from build123d import *

# Parameters (mm, degrees)
SKETCH_1_W               = 55
SKETCH_1_H               = 55
EXTRUDE_1_DEPTH          = 10
SKETCH_2_R               = 17.5
EXTRUDE_2_DEPTH          = 1
SKETCH_3_R               = 16.25
EXTRUDE_3_DEPTH          = 2
SKETCH_4_R               = 17.5
EXTRUDE_4_DEPTH          = 1
SKETCH_5_R               = 4.25
CUT_EXTRUDE_1_DEPTH      = 3
SKETCH_6_R               = 2.5
CUT_EXTRUDE_2_DEPTH      = 45.198416261
SKETCH_7_R               = 3.5
CUT_EXTRUDE_3_DEPTH      = 46.700109409
PATTERN_CIRCULAR_1_COUNT = 4
SKETCH_10_R              = 5
CUT_EXTRUDE_4_DEPTH      = 2
SKETCH_11_R              = 2
CUT_EXTRUDE_5_DEPTH      = 14
PATTERN_CIRCULAR_2_COUNT = 4
FILLET_1_R               = 1
CHAMFER_1_SIZE           = 0.5
CHAMFER_2_SIZE           = 1


with BuildPart() as part:
    # Sketch 1 → Extrude 1 (new, symmetric)
    with BuildSketch(Plane(origin=(0, 0, 0), x_dir=(1, 0, 0), z_dir=(0, 1, 0))):
        Rectangle(SKETCH_1_W, SKETCH_1_H)
    extrude(amount=EXTRUDE_1_DEPTH, both=True)

    # Sketch 2 → Extrude 2 (add)
    with BuildSketch(Plane(origin=(0, 10, 0), x_dir=(1, 0, 0), z_dir=(0, 1, 0))):
        with Locations(Location((0, 0, 0), (0, 0, 270))):
            Circle(SKETCH_2_R)
    extrude(amount=EXTRUDE_2_DEPTH)

    # Sketch 3 → Extrude 3 (add)
    with BuildSketch(Plane(origin=(0, 11, 0), x_dir=(1, 0, 0), z_dir=(0, 1, 0))):
        with Locations(Location((0, 0, 0), (0, 0, 270))):
            Circle(SKETCH_3_R)
    extrude(amount=EXTRUDE_3_DEPTH)

    # Sketch 4 → Extrude 4 (add)
    with BuildSketch(Plane(origin=(0, 13, 0), x_dir=(1, 0, 0), z_dir=(0, 1, 0))):
        with Locations(Location((0, 0, 0), (0, 0, 270))):
            Circle(SKETCH_4_R)
    extrude(amount=EXTRUDE_4_DEPTH)

    # Sketch 5 → Cut-Extrude 1 (cut)
    with BuildSketch(Plane.XZ.offset(10)):
        with Locations(Location((0, 20.75, 0), (0, 0, 270))):
            Circle(SKETCH_5_R)
    cut_extrude_1 = extrude(amount=-CUT_EXTRUDE_1_DEPTH, mode=Mode.SUBTRACT)

    # Sketch 6 → Cut-Extrude 2 (cut, through all)
    with BuildSketch(Plane.XZ.offset(7)):
        with Locations(Location((0, 20.75, 0), (0, 0, 270))):
            Circle(SKETCH_6_R)
    cut_extrude_2 = extrude(amount=-CUT_EXTRUDE_2_DEPTH, mode=Mode.SUBTRACT)

    # Sketch 7 → Cut-Extrude 3 (cut, through all)
    with BuildSketch(Plane.XZ.offset(10)):
        with Locations(Location((-22, 22, 0), (0, 0, 270))):
            Circle(SKETCH_7_R)
    cut_extrude_3 = extrude(amount=-CUT_EXTRUDE_3_DEPTH, mode=Mode.SUBTRACT)

    # Pattern Circular 1: Cut-Extrude 1, Cut-Extrude 2, Cut-Extrude 3 ×4 about axis
    pattern_circular_1_axis = Axis((0, 0, 0), (0, 1, 0))
    add([cut_extrude_1.rotate(pattern_circular_1_axis, i * 360 / PATTERN_CIRCULAR_1_COUNT) for i in range(1, PATTERN_CIRCULAR_1_COUNT)], mode=Mode.SUBTRACT)
    add([cut_extrude_2.rotate(pattern_circular_1_axis, i * 360 / PATTERN_CIRCULAR_1_COUNT) for i in range(1, PATTERN_CIRCULAR_1_COUNT)], mode=Mode.SUBTRACT)
    add([cut_extrude_3.rotate(pattern_circular_1_axis, i * 360 / PATTERN_CIRCULAR_1_COUNT) for i in range(1, PATTERN_CIRCULAR_1_COUNT)], mode=Mode.SUBTRACT)

    # Sketch 9 → M10x1.0 _1 (revolve, cut)
    with BuildSketch(Plane(origin=(-27.5, 0, -10.5), x_dir=(0, 0, 1), z_dir=(0, 1, 0))):
        Polygon((0, 0), (0, 24.703872786), (4.5, 22), (4.5, 0.525), (5.025, 0), align=None)
    m10x1_0_1 = revolve(axis=Axis((-33.85, 0, -10.5), (1, 0, 0)), mode=Mode.SUBTRACT)

    # Mirror 1: M10x1.0 _1 across plane
    add(m10x1_0_1.mirror(Plane(origin=(0, 0, 0), x_dir=(0, 0, 1), z_dir=(1, 0, 0))), mode=Mode.SUBTRACT)

    # Mirror 1 at the second plane: M10x1.0 _1 across plane
    add(m10x1_0_1.mirror(Plane.XY), mode=Mode.SUBTRACT)

    # Mirror 1 at the second plane copy 1 sket → Mirror 1 at the second plane copy 1 (revolve, cut)
    with BuildSketch(Plane(origin=(27.5, 0, 10.5), x_dir=(0, 0, -1), z_dir=(0, 1, 0))):
        Polygon((0, 0), (0, 24.703872786), (4.5, 22), (4.5, 0.525), (5.025, 0), align=None)
    revolve(axis=Axis((33.85, 0, 10.5), (-1, 0, 0)), mode=Mode.SUBTRACT)

    # Sketch 10 → Cut-Extrude 4 (cut)
    with BuildSketch(Plane(origin=(0, 14, 0), x_dir=(1, 0, 0), z_dir=(0, 1, 0))):
        with Locations(Location((0, 0, 0), (0, 0, 270))):
            Circle(SKETCH_10_R)
    extrude(amount=-CUT_EXTRUDE_4_DEPTH, mode=Mode.SUBTRACT)

    # Sketch 11 → Cut-Extrude 5 (cut)
    with BuildSketch(Plane(origin=(0, 14, 0), x_dir=(1, 0, 0), z_dir=(0, 1, 0))):
        with Locations(Location((7.778174593, 7.778174593, 0), (0, 0, 270))):
            Circle(SKETCH_11_R)
    cut_extrude_5 = extrude(amount=-CUT_EXTRUDE_5_DEPTH, mode=Mode.SUBTRACT)

    # Pattern Circular 2: Cut-Extrude 5 ×4 about axis
    pattern_circular_2_axis = Axis((0, 0, 0), (0, 1, 0))
    for i in range(1, PATTERN_CIRCULAR_2_COUNT):
        add(cut_extrude_5.rotate(pattern_circular_2_axis, i * 360 / PATTERN_CIRCULAR_2_COUNT), mode=Mode.SUBTRACT)

    # Fillet 1
    fillet_1_edges = [part.edges().sort_by_distance(p)[0] for p in [
        (27.5, 0, 27.5),
        (-27.5, 0, 27.5),
        (-27.5, 0, -27.5),
        (27.5, 0, -27.5),
    ]]
    fillet(fillet_1_edges, radius=FILLET_1_R)

    # Chamfer 1
    chamfer_1_edges = [part.edges().sort_by_distance(p)[0] for p in [
        (0, -10, 25),
        (-25, -10, 0),
        (0, -10, -25),
        (25, -10, 0),
    ]]
    chamfer(chamfer_1_edges, length=CHAMFER_1_SIZE)

    # Chamfer 2
    chamfer_2_edges = [part.edges().sort_by_distance(p)[0] for p in [
        (-22, -10, 25.5),
        (-25.5, -10, -22),
        (22, -10, -25.5),
        (25.5, -10, 22),
    ]]
    chamfer(chamfer_2_edges, length=CHAMFER_2_SIZE)


solid = part.part
Here's how the part is built. I have some questions about the finished solid (model axes, mm). A direction names the side the tool comes from. Coordinates: 2 decimals unless noted, no trailing zeros. Write each loop counter-clockwise with the first axis right and the second up, starting at its lowest first coordinate (ties: lowest second). Pieces come first, ordered by that corner, then holes.
Item 1: If we mould it in two halves opening along Y, with no side actions, what happens to faces 1 (the flat face through (2, -7, -19)), 2 (the cylindrical face through (23.248, 1.381, -0.11)), 3 (the cylindrical face through (-16.39, -3.04, -13.82)), 4 (the conical face through (3.266, -0.034, -11.281))? For each: +Y half, -Y half, draft (parallel to the pull), parting line (faces both ways), or undercut.
Item 2: On a 3-axis mill with a long thin cutter (end or side, diameter ignored), from which of +Z, -Z, +X, -X, +Y, -Y can I reach the whole of each face in a straight line? I mean faces 5 (the cylindrical face through (4.88, 11.99, 15.5)), 6 (the cylindrical face through (16.39, -3.04, -13.82)), 7 (the cylindrical face through (-8.212, 8.654, -5.826)), 8 (the cylindrical face through (24.12, -8.27, 2.59)), 9 (the cylindrical face through (-20.12, 0.37, -19.05)). Say none if no direction works.
Item 3: I want a section at B-B on x = -13.5. Write out the boundary of the cut face in (y, z), and give its area (3 significant figures).
Item 4: Will these pins go through, and if not, where does the flat tip stop? pin 1 (2.5 mm diameter, centred on x = 1, z = 22.5, fed in from -Y); pin 2 (5.5 mm diameter, centred on y = 0, z = -10.5, fed in from -X); pin 3 (5.5 mm diameter, centred on y = 0, z = -10.5, fed in from +X).
Item 5: I want a section at A-A on z = 0. Count the separate pieces of the cut face and the enclosed holes in it, and give its area (4 significant figures).
Item 6: If I drill on line 1 (Z direction, x = 15.5, y = 0); line 2 (X direction, y = 9, z = -8); line 3 (Y direction, x = -18.5, z = -10.5), over which ranges is the centre line in solid material (lowest first)?
Findings below:
1. face 1: -Y half
1. face 2: draft
1. face 3: undercut
1. face 4: undercut
2. face 5: none
2. face 6: +X
2. face 7: +Y
2. face 8: -Y
2. face 9: +Y, -Y
3. outline: (-10, -27.5) - (10, -27.5) - (10, -11.14) - (11, -11.14) - (11, -9.05) - (13, -9.05) - (13, -11.14) - (14, -11.14) - (14, 11.14) - (13, 11.14) - (13, 9.05) - (11, 9.05) - (11, 11.14) - (10, 11.14) - (10, 27.5) - (-10, 27.5) - close; hole circle Ø9 at (0, -10.5); hole circle Ø9 at (0, 10.5)
3. area: 1,050 mm2
4. pin 1: stops at y = -7
4. pin 2: stops at x = -4.45
4. pin 3: stops at x = 4.45
5. separate pieces: 3
5. enclosed holes: 0
5. area: 993.5 mm2
6. line 1: z = -27.5 to -15, -6 to 6, 15 to 27.5
6. line 2: x = -27.5 to -9.77, -5.79 to 5.79, 9.77 to 27.5
6. line 3: y = -10 to -4.5, 4.5 to 10
